CAD build for the part. Positions are in the model's coordinates, mm. A direction names the side the tool comes from. Round coordinates to 2 decimals unless told otherwise and drop trailing zeros. Order: outer loops, then holes, each group sorted by start corner. A loop starts at its lowest first (then second) coordinate and runs counter-clockwise, first axis right, second up. Notation, with made-up numbers: (0.25, 25.25) -> (4.25, 25.25) arc R21 cw to (4.25, 38.25) -> close; hole circle Ø9 at (-39, -21). An arc over 180 degrees is marked (long way). Return JSON: item names as keys, results as strings. Group by question number.
Q1. Cut at A-A (z = -17). Write the cut outline in (x, y), then the cut area to 3 significant figures.
Q2. Probe line 1 along Z through (x, y) = (1.25, -0.25); line 2 along Z through (x, y) = (3.25, 0); line 3 along Z through (x, y) = (1.5, -2.5). List the from-to ranges inside material, lowest first.
Q3. Which spindle directions (+Z, -Z, +X, -X, +Y, -Y) get a long thin tool onto all of the face, cutting with end or side? Do faces 5 (the cylindrical face through (3.1, -0.69, -32.63)), 6 (the flat face through (-1.984, 0, 35)), 7 (the flat face through (1.2, 2.2, 36.909)). Say none if no direction does.
Q4. Mould opens along X. For faces 1 (the flat face through (0, 0, -36.909)), 2 (the conical face through (1.06, -1.86, 36.76)), 3 (the cylindrical face through (0.166, -3.767, 30.186)), 4 (the flat face through (-0.978, 1.727, 34.855)) say: +X half, -X half, draft (parallel to the pull), parting line (faces both ways), or undercut.
Q5. Flat gauge pins, fed straight in: pin 1 (0.7 mm diameter, centred on y = -0.5, z = 34.5, fed in from -X); pin 2 (2 mm diameter, centred on x = -0.5, y = 4, fed in from -Z); pin 3 (1.5 mm diameter, centred on x = -2.5, y = -1.5, fed in from -Z); pin 4 (5 mm diameter, centred on x = 0, z = 17, fed in from -Y). Where does each tip first touch, or does it go through?
from build123d import *

# Parameters (mm, degrees)
CUT_EXTRUDE1_DEPTH = 4.1671875
SKETCH6_R          = 2.291358881
CUT_EXTRUDE4_DEPTH = 4.1671875
CUT_EXTRUDE4_DRAFT = -45


with BuildPart() as part:
    # Sketch4 → Revolve1 (revolve)
    with BuildSketch(Plane(origin=(0, 0, 0), x_dir=(0, 0, -1), z_dir=(1, 0, 0))):
        Polygon((-31.353125, 5.55625), (-36.35375, 5.55625), (-36.909375, 5.000625), (-36.909375, 0), (25.796875, 0), (25.796875, 3.704166667), (25.532291667, 3.96875), (-28.990925, 3.96875), (-29.1893625, 3.7703125), (-31.1546875, 3.7703125), (-31.353125, 3.96875), align=None)
    revolve(axis=Axis((0, 0, 36.909375), (0, 0, -1)))

    # Sketch5 → Cut-Extrude1 (cut)
    with BuildSketch(Plane.XY.offset(36.909375)):
        Polygon((1.984375, 1.14567944), (0, 2.291358881), (-1.984375, 1.14567944), (-1.984375, -1.14567944), (0, -2.291358881), (1.984375, -1.14567944), align=None)
    extrude(amount=-CUT_EXTRUDE1_DEPTH, mode=Mode.SUBTRACT)


with BuildPart() as cut_extrude4_tool:
    # Sketch6 → Cut-Extrude4 (with draft: the straight prism first)
    with BuildSketch(Plane.XY.offset(36.909375)):
        Circle(SKETCH6_R)
    extrude(amount=-CUT_EXTRUDE4_DEPTH)
    # Cut-Extrude4: the draft: its side faces are tilted about the plane it starts from
    cut_extrude4_sides = [cut_extrude4_tool.faces().sort_by_distance(p)[0] for p in [
        (-2.291358881, 0, 34.82578125),
    ]]
    draft(cut_extrude4_sides, Plane.XY.offset(36.909375), CUT_EXTRUDE4_DRAFT)


with BuildPart() as part_1:
    add(part.part)

    # Cut-Extrude4: cut by cut_extrude4_tool
    add(cut_extrude4_tool.part, mode=Mode.SUBTRACT)

    # Sketch7 → Revolve2 (revolve)
    with BuildSketch(Plane(origin=(0, 0, 0), x_dir=(0, 0, -1), z_dir=(1, 0, 0))):
        Polygon((25.796875, 3.175), (35.956875, 3.175), (36.909375, 2.2225), (36.909375, 0), (25.796875, 0), align=None)
    revolve(axis=Axis((0, 0, -36.909375), (0, 0, 1)))

    # Sketch10 → Cut-Revolve1 (revolve, cut)
    with BuildSketch(Plane(origin=(0, 0, 0), x_dir=(0, 0, -1), z_dir=(1, 0, 0))):
        with BuildLine():
            Line((26.660475, 2.3114), (28.336875, 2.3114))
            Line((28.336875, 2.3114), (29.994225, 3.96875))
            Line((29.994225, 3.96875), (25.796875, 3.96875))
            Line((25.796875, 3.96875), (25.796875, 3.175))
            ThreePointArc((25.796875, 3.175), (26.049817584, 2.564342584), (26.660475, 2.3114))
        make_face()
    revolve(axis=Axis((0, 0, -36.909375), (0, 0, 1)), mode=Mode.SUBTRACT)


solid = part_1.part
Solution:
{
 "1": {"outline": "circle Ø7.94 at (0, 0)", "area": "49.5 mm²"},
 "2": {"line 1": "z = -36.91 to 32.74", "line 2": "z = -25.8 to 36.91", "line 3": "z = -36.22 to -28.94, -25.84 to 36.91"},
 "3": {"face 5": "-Z", "face 6": "+Z", "face 7": "+Z, +X, -X, +Y, -Y"},
 "4": {"face 1": "draft", "face 2": "undercut", "face 3": "parting line", "face 4": "undercut"},
 "5": {"pin 1": "stops at x = -5.55", "pin 2": "stops at z = -36.1", "pin 3": "stops at z = -36.91", "pin 4": "stops at y = -3.97"}
}
